from build123d import *

# Parameters (mm, degrees)
SALIENTE_EXTRUIR1_DEPTH = 55
CORTAR_EXTRUIR1_DEPTH   = 68


with BuildPart() as part:
    # Croquis1 → Saliente-Extruir1 (new body)
    with BuildSketch(Plane.XY):
        Polygon((-7.08566541, -21.054004681), (20.287395509, -21.054004681), (-0.444607291, -12.379909579), (-6.980601691, -12.379909579), (-31.08566541, -21.054004681), align=None)
    extrude(amount=SALIENTE_EXTRUIR1_DEPTH)

    # Croquis2 → Cortar-Extruir1 (cut)
    with BuildSketch(Plane.XY):
        Polygon((-7.413108938, -12.812416826), (-0.041425498, -12.812416826), (1.379269414, -14.336446074), (1.379269414, -20.687882008), (-8.657749406, -20.687882008), (-8.657749406, -14.057057294), align=None)
    extrude(amount=CORTAR_EXTRUIR1_DEPTH, mode=Mode.SUBTRACT)


solid = part.part
Model file for the job. Use its own axes, mm. A direction names the side the tool comes from. Coordinates: 2 decimals unless noted, no trailing zeros. Write each loop counter-clockwise with the first axis right and the second up, starting at its lowest first coordinate (ties: lowest second). Pieces come first, ordered by that corner, then holes. Notation, with made-up numbers: (28.25, 88) - (60.25, 88) arc R21 ccw to (60.25, 120) - close; hole circle Ø7 at (67.25, -35). An arc over 180 degrees is marked (long way). Write each question's results on one line, items separated by ' | '. Start each with the question number.
1) Cut at B-B (z = 46). Write the cut outline in (x, y), then the cut area to 3 significant figures.
2) Mould opens along X. For faces 1 (the face through (-4, -12.812, 27)), 2 (the face through (-9, -19, 0)), 3 (the face through (-8.658, -17, 27)), 4 (the face through (10.07, -16.78, 27.12)) say: pulls with the +X half, pulls with the -X half, needs draft (parallel to the pull), parting line crosses it, or undercut.
3) 3-axis set-ups, long thin cutter, end or side, ignore diameter. For faces 5 (the face through (-18.864, -16.656, 27.115)), 6 (the face through (-4, -20.688, 27)): which of +Z, -Z, +X, -X, +Y, -Y reach the whole face in a straight line?
4) Probe line 1 along Y through (x, z) = (-6.5, 20); line 2 along Y through (x, z) = (-15, 21.5); line 3 along Y through (x, z) = (-12.5, 24). List the from-to ranges inside material, lowest first. Write a range as from..to.
5) Cut at A-A (y = -15). Write the cut outline in (x, z), then the cut area to 3 significant figures.
6) Cut at C-C (x = 15). Write the cut outline in (y, z).
7) Flat gauge pins, fed straight in: P1, Ø2, axis at y = -16.5, z = 21, coming from the +X side; P2, Ø12, axis at x = -13.5, z = 30.5, coming from the +Y side. Where does each tip first touch, or does it go through?
8) Cut at D-D (y = -20). Write the cut outline in (x, z), then the cut area to 3 significant figures.
Returned:
1) outline: (-31.09, -21.05) - (20.29, -21.05) - (-0.44, -12.38) - (-6.98, -12.38) - close; hole (-8.66, -20.69) - (1.38, -20.69) - (1.38, -14.34) - (-0.04, -12.81) - (-7.41, -12.81) - (-8.66, -14.06) - close | area: 174 mm^2
2) face 1: undercut | face 2: needs draft | face 3: undercut | face 4: pulls with the +X half
3) face 5: +Z, -Z, -X, +Y | face 6: +Z, -Z
4) line 1: -21.05..-20.69, -12.81..-12.38 | line 2: -21.05..-15.27 | line 3: -21.05..-14.37
5) outline: (-14.26, 0) - (-8.66, 0) - (-8.66, 55) - (-14.26, 55) - close; (1.38, 0) - (5.82, 0) - (5.82, 55) - (1.38, 55) - close | area: 552 mm^2
6) outline: (-21.05, 0) - (-18.84, 0) - (-18.84, 55) - (-21.05, 55) - close
7) P1: x = 11.79 | P2: y = -12.57
8) outline: (-28.16, 0) - (-8.66, 0) - (-8.66, 55) - (-28.16, 55) - close; (1.38, 0) - (17.77, 0) - (17.77, 55) - (1.38, 55) - close | area: 1,970 mm^2
